```python
from build123d import *

# Parameters (mm, degrees)
SKETCH2_R               = 1.5
CUT_EXTRUDE1_DEPTH      = 10
CUT_EXTRUDE2_DEPTH      = 10
CUT_EXTRUDE2_DEPTH_BACK = 10
SKETCH3_W               = 11.471414326
SKETCH3_H               = 1.059782784


with BuildPart() as part:
    # Sketch1 → Revolve1 (revolve)
    with BuildSketch(Plane(origin=(0, 0, 0), x_dir=(0, 0, -1), z_dir=(1, 0, 0)), mode=Mode.PRIVATE) as revolve1_sk:
        with BuildLine():
            Line((0, 8.65), (0, 0))
            Line((0, 0), (3.2, 0))
            Line((3.2, 0), (3.2, 1))
            Line((3.2, 1), (1.8, 1.808290377))
            Line((1.8, 1.808290377), (1.8, 2.693988174))
            ThreePointArc((1.8, 2.693988174), (3.111031857, 6.340202523), (0, 8.65))
        make_face()
    revolve(revolve1_sk.sketch.rotate(Axis((0, 8.65, 0), (0, -1, 0)), 180), axis=Axis((0, 8.65, 0), (0, -1, 0)))

    # Sketch2 → Cut-Extrude1 (cut)
    with BuildSketch(Plane.XZ):
        with Locations(Location((0, 0, 0), (0, 0, 270))):
            Circle(SKETCH2_R)
    extrude(amount=-CUT_EXTRUDE1_DEPTH, mode=Mode.SUBTRACT)

    # Sketch3 → Cut-Extrude2 (cut, two sides: drawn at the far end of the back side and taken through both)
    with BuildSketch(Plane(origin=(0, 0, 0), x_dir=(0, 0, -1), z_dir=(1, 0, 0)).offset(-CUT_EXTRUDE2_DEPTH_BACK)):
        with Locations((2.521032719, 8.529891392)):
            Rectangle(SKETCH3_W, SKETCH3_H)
    extrude(amount=CUT_EXTRUDE2_DEPTH + CUT_EXTRUDE2_DEPTH_BACK, mode=Mode.SUBTRACT)


solid = part.part
```
Geometry check sheet. Reference: the model listing, model coordinates, mm. Give positions to 0.01 mm unless a question says otherwise; leave off trailing zeros. Order: outer loops, then holes, each group sorted by start corner. A loop starts at its lowest first (then second) coordinate and runs counter-clockwise, first axis right, second up.
1. Section check C-C, the plane y = 7. Enter the section's corners in (x, z), and give its area (3 significant figures).
2. Gauge pin test, flat ends, axial feed: pin 1 Ø3 at (x, z) = (-2, 1.5) entering from +Y; pin 2 Ø1 at (y, z) = (6, 0.5) entering from -X. Record the tip position at first contact, or that the pin passes through.
3. Section check B-B, the plane y = 3.75. Enter the section's corners in (x, z).
4. Thickness scan on L1, parallel to X at y = 4, z = 0; L2, parallel to Y at x = -2.75, z = -1; L3, parallel to Y at x = -2.25, z = -0.75. Record the ranges inside material, lowest first.
5. Release check for a two-part mould opening along Y. For faces 1 (the face through (-0.541, 2.257, 1.717)), 2 (the face through (-1.5, 0, -0.7)), 3 (the face through (0.45, 3.94, -1.43)) record: pulls with the +Y half, pulls with the -Y half, needs draft (parallel to the pull), parting line crosses it, or undercut.
6. Section check A-A, the plane z = 0. Enter the section's corners in (x, y).
Values follow:
1. outline: circle Ø5.66 at (0, 0); hole circle Ø3 at (0, 0)
1. area: 18.1 mm2
2. pin 1: stops at y = 8
2. pin 2: stops at x = -3.24
3. outline: circle Ø5.6 at (0, 0); hole circle Ø3 at (0, 0)
4. L1: x = -2.93 to -1.5, 1.5 to 2.93
4. L2: y = 0 to 1.16, 3.99 to 6.81
4. L3: y = 0 to 1.48, 3.18 to 7.62
5. face 1: undercut
5. face 2: pulls with the -Y half
5. face 3: needs draft
6. outline: (-3.2, 0) - (-1.5, 0) - (-1.5, 8) - (-1.95, 8) arc R3.25 ccw to (-1.8, 2.69) - (-1.8, 1.81) - (-3.2, 1) - close; (1.5, 0) - (3.2, 0) - (3.2, 1) - (1.8, 1.81) - (1.8, 2.69) arc R3.25 ccw to (1.95, 8) - (1.5, 8) - close
